Design review of the part built by this model. Coordinates are the model's own, in mm. Round coordinates to 2 decimals unless told otherwise and drop trailing zeros. Order: outer loops, then holes, each group sorted by start corner. A loop starts at its lowest first (then second) coordinate and runs counter-clockwise, first axis right, second up. Notation, with made-up numbers: M 11.25,82 L 59.25,82 A21 ccw 59.25,115 Z; hole C 59,-18.5 d6. An arc over 180 degrees is marked long. Use a Markdown table: item, result. Add a question column.
(1) To check wall thickness, follow probe 1 along Y at (x, z) = (0, 2.85) (1 decimal); probe 2 along X at (y, z) = (-13, 2.9); probe 3 along X at (y, z) = (-5, 1.45). State the ranges of each line that lie inside material, in increasing order. Write a range as from..to.
(2) Take a section at C-C (x = -9). Write out the cut boundary in (y, z), then the cut area to 3 significant figures.
(3) The part is to be moulded in two halves that separate along X. For faces 1 (the face through (17.847, 1, 3)), 2 (the face through (8.64, -6.34, 2.5)), 3 (the face through (4, 1, 0)), 4 (the face through (-16.687, -19.858, 2.576)), say which applies: released by +X, released by -X, zero draft, split by the parting line, or undercut.
(4) Take a section at A-A (y = 0). Write out the cut boundary in (x, z) (3 decimals).
(5) Take a section at B-B (x = 0). Write out the cut boundary in (y, z) (1 decimal).
(6) Take a section at D-D (y = 15). Write out the cut boundary in (x, z).
(7) For pin 1 (4 mm diameter, centred on x = 0, y = 10.165, fed in from -Z), flat-tipped, find the tip position at first contact; note if it passes through.
Autodesk Inventor part; units mm, degrees
ref_plane "YZ Plane" through (0, 0, 0) normal (1, 0, 0) x (0, 1, 0)
ref_plane "XZ Plane" through (0, 0, 0) normal (0, 1, 0) x (-1, 0, 0)
ref_plane "XY Plane" through (0, 0, 0) normal (0, 0, 1) x (1, 0, 0)
sketch "Sketch1" plane through (0, 0, 0) normal (0, 0, 1) x (1, 0, 0)
  circle A0 centre (-9.6692, -12.9185) radius 3.175
  circle A1 centre (9.3808, -12.9185) radius 3.175
  circle A2 centre (9.3808, 14.1748) radius 3.175
  circle A3 centre (-9.6692, 14.1748) radius 3.175
  line L0 (-9.6692, 14.1748) -> (9.3808, 14.1748) construction
  line L1 (9.3808, 14.1748) -> (9.3808, -12.9185) construction
  line L2 (9.3808, -12.9185) -> (-9.6692, -12.9185) construction
  line L3 (-9.6692, -12.9185) -> (-9.6692, 14.1748) construction
  line L4 (-18.1359, 22.6415) -> (17.8474, 22.6415)
  line L5 (17.8474, 22.6415) -> (17.8474, -21.3852)
  line L6 (17.8474, -21.3852) -> (-18.1359, -21.3852)
  line L7 (-18.1359, -21.3852) -> (-18.1359, 22.6415)
  circle A4 centre (0, 0) radius 10.165 construction
  circle A5 centre (0, 10.165) radius 1.27
  circle A6 centre (-8.8031, 5.0825) radius 1.27
  circle A7 centre (-8.8031, -5.0825) radius 1.27
  circle A8 centre (0, -10.165) radius 1.27
  circle A9 centre (8.8031, -5.0825) radius 1.27
  circle A10 centre (8.8031, 5.0825) radius 1.27
  dimension "d7" = 20.3299
  dimension "d0" = 8.4667
  dimension "d1" = 8.4667
  dimension "d2" = 8.4667
  dimension "d3" = 8.4667
  dimension "d4" = 6.35
  dimension "d8" = 2.54
  dimension "d11" = 360
extrude "Plate2" add sketch "Sketch1" along normal blind 5.08
fillet "Fillet1" radius 5.08 4 edges at (-18.1359, -21.3852, 2.54) (17.8474, -21.3852, 2.54) (17.8474, 22.6415, 2.54) (-18.1359, 22.6415, 2.54)
sketch "Sketch4" plane through (0, 0, 5.08) normal (0, 0, 1) x (1, 0, 0)
  point P0 (0, 0)
hole "Hole1" at (0, 0, 5.08) direction (0, 0, -1) diameter 6.35 end through all
equation "\"d18\" = Thickness"
equation "\"d5\" = Thickness"
equation "\"BendRadius\" = Thickness"
equation "\"BendReliefWidth\" = Thickness"
equation "\"BendReliefDepth\" = 0.5 * Thickness"
equation "\"CornerReliefSize\" = 4 * Thickness"
equation "\"MinimumRemnant\" = 2 * Thickness"
equation "\"TransitionRadius\" = BendRadius"
equation "\"JacobiRadiusSize\" = BendRadius"
equation "\"GapSize\" = Thickness"
properties part number "UpperArmShoulderMount"
Verdict:
| question | item | result |
|---|---|---|
| 1 | probe 1 | y = -21.4..-11.4, -8.9..-3.2, 3.2..8.9, 11.4..22.6 |
| 1 | probe 2 | x = -18.14..-12.84, -6.5..6.21, 12.55..17.85 |
| 1 | probe 3 | x = -18.14..-10.07, -7.54..7.54, 10.07..17.85 |
| 2 | outline | M -21.39,0 L -16.02,0 L -16.02,5.08 L -21.39,5.08 Z; M -9.81,0 L -6.34,0 L -6.34,5.08 L -9.81,5.08 Z; M -3.83,0 L 3.83,0 L 3.83,5.08 L -3.83,5.08 Z; M 6.34,0 L 11.07,0 L 11.07,5.08 L 6.34,5.08 Z; M 17.28,0 L 22.64,0 L 22.64,5.08 L 17.28,5.08 Z |
| 2 | area | 135 mm^2 |
| 3 | face 1 | released by +X |
| 3 | face 2 | undercut |
| 3 | face 3 | zero draft |
| 3 | face 4 | released by -X |
| 4 | outline | M -18.136,0 L -3.175,0 L -3.175,5.08 L -18.136,5.08 Z; M 3.175,0 L 17.847,0 L 17.847,5.08 L 3.175,5.08 Z |
| 5 | outline | M -21.4,0 L -11.4,0 L -11.4,5.1 L -21.4,5.1 Z; M -8.9,0 L -3.2,0 L -3.2,5.1 L -8.9,5.1 Z; M 3.2,0 L 8.9,0 L 8.9,5.1 L 3.2,5.1 Z; M 11.4,0 L 22.6,0 L 22.6,5.1 L 11.4,5.1 Z |
| 6 | outline | M -18.14,0 L -12.74,0 L -12.74,5.08 L -18.14,5.08 Z; M -6.6,0 L 6.31,0 L 6.31,5.08 L -6.6,5.08 Z; M 12.45,0 L 17.85,0 L 17.85,5.08 L 12.45,5.08 Z |
| 7 | pin 1 | stops at z = 0 |
